Design review of the part built by this model. Coordinates are the model's own, in mm. Face numbers are marked on the shaded views. Coordinates: 2 decimals unless noted, no trailing zeros. Loops run counter-clockwise (first coordinate to the right, second up) from the corner with the lowest first, then second, coordinate; pieces in that order, holes last. Notation, with made-up numbers: M -22.75,28.5 L 12.25,28.5 A19 cw 12.25,61.5 Z; hole C -37.5,-11 d4. An arc over 180 degrees is marked long. Answer as a JSON object with one key per item and string values. Group by question number.
1. Draft analysis for pull direction X (two halves, no side actions). For the marked faces 1, 2 and 3, state which applies: +X half, -X half, draft (parallel to the pull), parting line (faces both ways), or undercut.
2. Consider section D-D (y = 0). State the section outline as (x, z) points, then the cut area to 3 significant figures.
3. Consider section B-B (x = 0). State the section outline as (y, z) points, then the cut area to 3 significant figures.
4. Consider section A-A (z = 12). State the section outline as (x, y) points, then the cut area to 3 significant figures.
5. Insertion check: pin 1 (1.5 mm diameter, centred on x = -258, z = -44, fed in from +Y); pin 2 (3 mm diameter, centred on y = 153, z = -56.5, fed in from -X); pin 3 (6.5 mm diameter, centred on y = 156.5, z = -49, fed in from +X). Each pin has a flat end and moves straight along its axis. Give the tip position at first contact, or say it passes through.
6. To check wall thickness, follow probe 1 along Y at (x, z) = (0, 25); probe 2 along Y at (x, z) = (-320, -52); probe 3 along X at (y, z) = (162.5, -62.5). State the ranges of each line that lie inside material, in increasing order.
7. Consider section C-C (y = 152.4). State the section outline as (x, z) points, then the cut area to 3 significant figures.
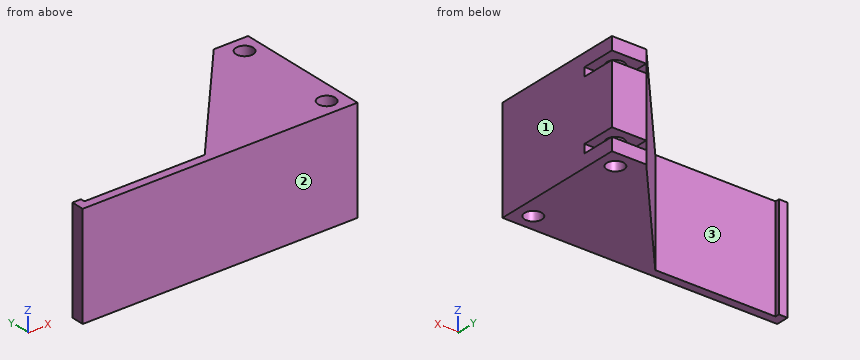
from build123d import *

# Parameters (mm, degrees)
SKETCH1_W               = 381
SKETCH1_H               = 25.4
SKETCH1_W_2             = 25.4
SKETCH1_H_2             = 152.4
BOSS_EXTRUDE1_DEPTH     = 76.2
CUT_EXTRUDE1_DEPTH      = 470.041106941
CUT_EXTRUDE1_DEPTH_BACK = 470.041106941
SKETCH2_R               = 12.7
SKETCH4_W               = 50.8
SKETCH4_H               = 50.8
CUT_EXTRUDE2_DEPTH      = 6.35
CUT_EXTRUDE3_DEPTH      = 451.089146725
CUT_EXTRUDE3_DEPTH_BACK = 451.089146725
SKETCH5_W               = 381
SKETCH5_H               = 25.4
BOSS_EXTRUDE2_DEPTH     = 76.2


with BuildPart() as part:
    # Sketch1 → Boss-Extrude1 (new, symmetric)
    with BuildSketch(Plane.XY):
        with Locations((-215.9, 12.7)):
            Rectangle(SKETCH1_W, SKETCH1_H)
        with Locations((-12.7, 76.2)):
            Rectangle(SKETCH1_W_2, SKETCH1_H_2)
        Polygon((0, 152.4), (0, 0), (-25.4, 0), (-25.4, -25.4), (25.4, -25.4), (25.4, 177.8), (-25.4, 177.8), (-25.4, 152.4), align=None)
    extrude(amount=BOSS_EXTRUDE1_DEPTH, both=True)

    # Sketch2 → Cut-Extrude1 (cut, two sides: drawn at the far end of the back side and taken through both)
    with BuildSketch(Plane.XY.offset(76.2).offset(-CUT_EXTRUDE1_DEPTH_BACK)):
        Circle(SKETCH2_R)
        with Locations((0, 152.4)):
            Circle(SKETCH2_R)
    extrude(amount=CUT_EXTRUDE1_DEPTH + CUT_EXTRUDE1_DEPTH_BACK, mode=Mode.SUBTRACT)

    # Sketch4 → Cut-Extrude2 (cut, symmetric)
    with BuildSketch(Plane.XY.offset(50.8)):
        with Locations((0, 152.4)):
            Rectangle(SKETCH4_W, SKETCH4_H)
    cut_extrude2 = extrude(amount=CUT_EXTRUDE2_DEPTH, both=True, mode=Mode.SUBTRACT)

    # Mirror1: Cut-Extrude2 across plane
    add(cut_extrude2.mirror(Plane.XY), mode=Mode.SUBTRACT)

    # Sketch5 → Cut-Extrude3 (cut, two sides: drawn at the far end of the back side and taken through both)
    with BuildSketch(Plane.XY.offset(-CUT_EXTRUDE3_DEPTH_BACK)):
        with Locations((-215.9, 12.7)):
            Rectangle(SKETCH5_W, SKETCH5_H)
    extrude(amount=CUT_EXTRUDE3_DEPTH + CUT_EXTRUDE3_DEPTH_BACK, mode=Mode.SUBTRACT)

    # Sketch6 → Boss-Extrude2 (add, symmetric)
    with BuildSketch(Plane.XY):
        Polygon((-25.4, -25.4), (-381, -25.4), (-381, -6.35), (-368.3, -6.35), (-368.3, -12.7), (-190.5, -12.7), (-25.4, 177.8), align=None)
    extrude(amount=BOSS_EXTRUDE2_DEPTH, both=True)


solid = part.part
Findings below:
{
 "1": {"face 1": "+X half", "face 2": "draft", "face 3": "undercut"},
 "2": {"outline": "M -179.49,-76.2 L -12.7,-76.2 L -12.7,76.2 L -179.49,76.2 Z; M 12.7,-76.2 L 25.4,-76.2 L 25.4,76.2 L 12.7,76.2 Z", "area": "27,400 mm^2"},
 "3": {"outline": "M -25.4,-76.2 L -12.7,-76.2 L -12.7,76.2 L -25.4,76.2 Z; M 12.7,-76.2 L 139.7,-76.2 L 139.7,-57.15 L 127,-57.15 L 127,-44.45 L 139.7,-44.45 L 139.7,44.45 L 127,44.45 L 127,57.15 L 139.7,57.15 L 139.7,76.2 L 12.7,76.2 Z; M 165.1,-76.2 L 177.8,-76.2 L 177.8,-57.15 L 165.1,-57.15 Z; M 165.1,-44.45 L 177.8,-44.45 L 177.8,44.45 L 165.1,44.45 Z; M 165.1,57.15 L 177.8,57.15 L 177.8,76.2 L 165.1,76.2 Z", "area": "22,600 mm^2"},
 "4": {"outline": "M -381,-25.4 L 25.4,-25.4 L 25.4,177.8 L -25.4,177.8 L -190.5,-12.7 L -368.3,-12.7 L -368.3,-6.35 L -381,-6.35 Z; hole C 0,0 d25.4; hole C 0,152.4 d25.4", "area": "29,600 mm^2"},
 "5": {"pin 1": "stops at y = -12.7", "pin 2": "stops at x = -48.19", "pin 3": "stops at x = -25.4"},
 "6": {"probe 1": "y = -25.4 to -12.7, 12.7 to 139.7, 165.1 to 177.8", "probe 2": "y = -25.4 to -12.7", "probe 3": "x = -38.66 to -7.7, 7.7 to 25.4"},
 "7": {"outline": "M -47.41,-76.2 L -12.7,-76.2 L -12.7,-57.15 L -25.4,-57.15 L -25.4,-44.45 L -12.7,-44.45 L -12.7,44.45 L -25.4,44.45 L -25.4,57.15 L -12.7,57.15 L -12.7,76.2 L -47.41,76.2 Z; M 12.7,-76.2 L 25.4,-76.2 L 25.4,-57.15 L 12.7,-57.15 Z; M 12.7,-44.45 L 25.4,-44.45 L 25.4,44.45 L 12.7,44.45 Z; M 12.7,57.15 L 25.4,57.15 L 25.4,76.2 L 12.7,76.2 Z", "area": "6,580 mm^2"}
}
